Geometry: final body of the model. Coordinates: model frame, mm. A direction names the side the tool comes from. Coordinates: 2 decimals unless noted, no trailing zeros. Loops run counter-clockwise (first coordinate to the right, second up) from the corner with the lowest first, then second, coordinate; pieces in that order, holes last. Notation, with made-up numbers: (-35, -17.5) - (-16, -17.5) arc R24 ccw to (-16, -6.5) - close; hole circle Ø7 at (13, 62). An arc over 180 degrees is marked (long way). Write each question's results on one line, items separated by ' | '. Start each with the question number.
from build123d import *

# Parameters (mm, degrees)
BOSS_EXTRUDE1_DEPTH = 10
SKETCH2_W           = 10
SKETCH2_H           = 4
BOSS_EXTRUDE2_DEPTH = 5
SKETCH3_W           = 10
SKETCH3_H           = 7.5
BOSS_EXTRUDE3_DEPTH = 10
CHAMFER1_SIZE       = 5
SKETCH4_W           = 3
SKETCH4_H           = 1
CUT_EXTRUDE1_DEPTH  = 10


with BuildPart() as part:
    # Sketch1 → Boss-Extrude1 (new body)
    with BuildSketch(Plane(origin=(0, 0, 0), x_dir=(0, 0, -1), z_dir=(1, 0, 0))):
        Polygon((-22.923508233, 18.622830226), (-22.923508233, -36.377169774), (67.076491767, -36.377169774), (77.076491767, -26.377169774), (77.076491767, 13.622830226), (65.041232226, 23.622830226), (-14.958767774, 23.622830226), align=None)
    extrude(amount=-BOSS_EXTRUDE1_DEPTH)

    # Sketch2 → Boss-Extrude2 (add)
    with BuildSketch(Plane.XY.offset(22.923508233)):
        with Locations((-5, 2.622830226)):
            Rectangle(SKETCH2_W, SKETCH2_H)
    extrude(amount=BOSS_EXTRUDE2_DEPTH)

    # Sketch3 → Boss-Extrude3 (add, symmetric)
    with BuildSketch(Plane.XY.offset(22.923508233)):
        with Locations((-5, 19.872830226)):
            Rectangle(SKETCH3_W, SKETCH3_H)
    extrude(amount=BOSS_EXTRUDE3_DEPTH, both=True)

    # Chamfer1
    chamfer1_edges = [part.edges().sort_by_distance(p)[0] for p in [
        (-5, 23.622830226, 32.923508233),
    ]]
    chamfer(chamfer1_edges, length=CHAMFER1_SIZE)

    # Sketch4 → Cut-Extrude1 (cut)
    with BuildSketch(Plane(origin=(0, 0, 0), x_dir=(0, 0, -1), z_dir=(1, 0, 0))):
        with Locations((-26.423508233, 2.222830226)):
            Rectangle(SKETCH4_W, SKETCH4_H)
    extrude(amount=-CUT_EXTRUDE1_DEPTH, mode=Mode.SUBTRACT)


solid = part.part
1) Access query for faces 1 (the flat face through (-5, 17, 32.924)), 2 (the flat face through (-5, 16.123, 28)), 3 (the flat face through (-5, 4, 27.924)). Directions: +Z, -Z, +X, -X, +Y, -Y. A direction counts if a zero-diameter tool reaches every point of the face in a straight line with its end or side. Return the directions, or none.
2) Pin query (flat end, axial travel): pin 1 Ø5 at (x, y) = (-8, 8) entering from +Z; pin 2 Ø3 at (x, z) = (-3.5, 26) entering from -Y; pin 3 Ø0.6 at (x, y) = (-6.5, 4) entering from +Z. Return the tip coordinate at first contact, or that it passes through.
3) Section query B-B on y = -17.5. Output: boundary loops of the cut face in (x, z).
4) Material intervals for line 1 (Y direction, x = -1, z = 27.5); line 2 (Z direction, x = -3.5, y = -20); line 3 (Y direction, x = -2.5, z = 24.5), sorted ascending. Write a range as [from, to].
5) Section query A-A on x = -7. Output: boundary loops of the cut face in (y, z), and give its area (3 significant figures).
6) Pull-direction query (Y, two-part tool) for faces 4 (the flat face through (-5, 0.623, 25)), 5 (the flat face through (0, -6, -21)), 6 (the flat face through (-5, 1.723, 26)); classes: released by +Y, released by -Y, zero draft, split by the parting line, or undercut.
Returned:
1) face 1: +Z, +X, -X, +Y, -Y | face 2: +Z, +X, -X | face 3: +Z, +X, -X, -Y
2) pin 1: stops at z = 22.92 | pin 2: stops at y = 0.62 | pin 3: stops at z = 27.92
3) outline: (-10, -77.08) - (0, -77.08) - (0, 22.92) - (-10, 22.92) - close
4) line 1: y = [0.62, 1.72], [2.72, 4.62], [16.12, 23.62] | line 2: z = [-77.08, 22.92] | line 3: y = [0.62, 4.62], [16.12, 23.62]
5) outline: (-36.38, -67.08) - (-26.38, -77.08) - (13.62, -77.08) - (23.62, -65.04) - (23.62, 27.92) - (18.62, 32.92) - (16.12, 32.92) - (16.12, 22.92) - (4.62, 22.92) - (4.62, 27.92) - (2.72, 27.92) - (2.72, 24.92) - (1.72, 24.92) - (1.72, 27.92) - (0.62, 27.92) - (0.62, 22.92) - (-36.38, 22.92) - close | area: 5,970 mm²
6) face 4: released by -Y | face 5: zero draft | face 6: undercut
